The model under review builds one solid part; all positions refer to its coordinate system, in mm. A direction names the side the tool comes from. Coordinates: 2 decimals unless noted, no trailing zeros. Order: outer loops, then holes, each group sorted by start corner. A loop starts at its lowest first (then second) coordinate and runs counter-clockwise, first axis right, second up. Notation, with made-up numbers: M 63.5,24.5 L 87.5,24.5 A11 cw 87.5,38.5 Z; hole C 87,-11 d1. An arc over 180 degrees is marked long. Answer in a Markdown table with one row per item.
from build123d import *

# Parameters (mm, degrees)
PAD_DEPTH       = 0.25
SKETCH001_R     = 1.675
POCKET_DEPTH    = 5
SKETCH002_R     = 1.68
PAD001_DEPTH    = 0.85
SKETCH003_R     = 1.5
POCKET001_DEPTH = 0.75
FILLET_R        = 0.3
FILLET001_R     = 0.5
FILLET002_R     = 0.5
SKETCH004_W     = 0.25
SKETCH004_H     = 7.75
PAD002_DEPTH    = 2.5
SKETCH005_R     = 0.5
POCKET002_DEPTH = 5
FILLET003_R     = 0.2
PAD003_DEPTH    = 0.25


with BuildPart() as part:
    # Sketch → Pad (new body)
    with BuildSketch(Plane.XY):
        with BuildLine():
            ThreePointArc((-3.35, 0), (0, -3.35), (3.35, 0))
            Line((3.35, 8.75), (3.35, 0))
            Line((-3.35, 8.75), (3.35, 8.75))
            Line((-3.35, 0), (-3.35, 8.75))
        make_face()
    extrude(amount=PAD_DEPTH)

    # Sketch001 → Pocket (cut)
    with BuildSketch(Plane.XY):
        Circle(SKETCH001_R)
    extrude(amount=POCKET_DEPTH, mode=Mode.SUBTRACT)

    # Sketch002 (on DatumPlane) → Pad001 (join)
    with BuildSketch(Plane.XY.offset(0.85)):
        Circle(SKETCH002_R)
    extrude(amount=-PAD001_DEPTH)

    # Sketch003 → Pocket001 (cut)
    with BuildSketch(Plane.XY):
        Circle(SKETCH003_R)
    extrude(amount=POCKET001_DEPTH, mode=Mode.SUBTRACT)

    # Fillet
    fillet_edges = [part.edges().sort_by_distance(p)[0] for p in [
        (-1.68, 0, 0.85),
    ]]
    fillet(fillet_edges, radius=FILLET_R)

    # Fillet001
    fillet001_edges = [part.edges().sort_by_distance(p)[0] for p in [
        (-1.68, 0, 0.25),
    ]]
    fillet(fillet001_edges, radius=FILLET001_R)

    # Fillet002
    fillet002_edges = [part.edges().sort_by_distance(p)[0] for p in [
        (-1.5, 0, 0.75),
    ]]
    fillet(fillet002_edges, radius=FILLET002_R)

    # Sketch004 → Pad002 (join, symmetric)
    with BuildSketch(Plane.YZ):
        with Locations((8.625, -3.625)):
            Rectangle(SKETCH004_W, SKETCH004_H)
    extrude(amount=PAD002_DEPTH, both=True)

    # Sketch005 (on DatumPlane) → Pocket002 (cut)
    with BuildSketch(Plane.XZ.offset(-8.75)):
        with Locations((-1.5, -1.5)):
            Circle(SKETCH005_R)
        with Locations((-1.5, -6.5)):
            Circle(SKETCH005_R)
        with BuildLine():
            ThreePointArc((0, -7), (-0.353553, -7.146447), (-0.5, -7.5))
            Line((-0.5, -7.5), (0, -7.5))
            Line((0, -7), (0, -7.5))
        make_face()
    pocket002 = extrude(amount=POCKET002_DEPTH, mode=Mode.SUBTRACT)

    # Mirrored: Pocket002 across Sketch005 V_Axis
    add(pocket002.mirror(Plane(origin=(0, 8.75, 0), x_dir=(0, -1, 0), z_dir=(1, 0, 0))), mode=Mode.SUBTRACT)

    # Fillet003
    fillet003_edges = [part.edges().sort_by_distance(p)[0] for p in [
        (0, 8.75, 0.25),
    ]]
    fillet(fillet003_edges, radius=FILLET003_R)

    # Sketch006 (on DatumPlane) → Pad003 (join)
    with BuildSketch(Plane.XZ.offset(-8.75)):
        Polygon((-2.433517, -0.657248), (-3.325729, 0), (-2.433517, 0), align=None)
    pad003 = extrude(amount=PAD003_DEPTH)

    # Mirrored001: Pad003 across Sketch006 V_Axis
    add(pad003.mirror(Plane(origin=(0, 8.75, 0), x_dir=(0, -1, 0), z_dir=(1, 0, 0))))


solid = part.part
(1) Take a section at D-D (z = -5.25). Write out the cut boundary in (x, y), then the cut area to 3 significant figures.
Report:
| item | result |
|---|---|
| outline | M -2.5,8.5 L 2.5,8.5 L 2.5,8.75 L -2.5,8.75 Z |
| area | 1.25 mm^2 |
(2) Take a section at B-B (y = 7.5). Write out the cut boundary in (x, z), then the cut area to 4 significant figures.
Report:
| item | result |
|---|---|
| outline | M -3.35,0 L 3.35,0 L 3.35,0.25 L -3.35,0.25 Z |
| area | 1.675 mm^2 |
(3) Insertion check: P1, Ø0.6, axis at x = 0, y = -0.5, coming from the -Z side; P2, Ø3, axis at x = -1, y = -2, coming from the +Z side; P3, Ø2, axis at y = -1.5, z = -2.5, coming from the +X side; P4, Ø1, axis at x = -1, y = -1, coming from the -Z side. Each pin has a flat end and moves straight along its axis. Give the tip position at first contact, or say it passes through.
Report:
| item | result |
|---|---|
| P1 | z = 0.75 |
| P2 | z = 0.85 |
| P3 | through |
| P4 | z = 0 |
(4) Take a section at A-A (z = -1.5). Write out the cut boundary in (x, y), then the cut area to 3 significant figures.
Report:
| item | result |
|---|---|
| outline | M -2.5,8.5 L -2,8.5 L -2,8.75 L -2.5,8.75 Z; M -1,8.5 L 1,8.5 L 1,8.75 L -1,8.75 Z; M 2,8.5 L 2.5,8.5 L 2.5,8.75 L 2,8.75 Z |
| area | 0.750 mm^2 |
(5) To check wall thickness, follow line 1 (Z direction, x = 1.5, y = 8.6); line 2 (Y direction, x = 1.5, z = -0.25); line 3 (Z direction, x = -2, y = 2.5). State the ranges of each line that lie inside material, in increasing order. Write a range as [from, to].
Report:
| item | result |
|---|---|
| line 1 | [-7.5, -7], [-6, -2], [-1, 0.24] |
| line 2 | [8.5, 8.75] |
| line 3 | [0, 0.25] |
(6) Machinability: for faces 1 (the flat face through (0, 8.5, -4)), 2 (the flat face through (0, 8.75, -4)), which of the approach directions +Z, -Z, +X, -X, +Y, -Y give a long, thin tool a straight path to every point of the face, cutting with its end or side? Answer none if there is none.
Report:
| item | result |
|---|---|
| face 1 | -Z, +X, -X, -Y |
| face 2 | +Z, -Z, +X, -X, +Y |
(7) Take a section at C-C (x = 3). Write out the cut boundary in (y, z).
Report:
| item | result |
|---|---|
| outline | M -1.49,0 L 8.5,0 L 8.5,-0.24 L 8.75,-0.24 L 8.75,0.05 A0.2 ccw 8.55,0.25 L -1.49,0.25 Z |
